Verification items for the finished model (mm, model axes). A direction names the side the tool comes from. Round coordinates to 2 decimals unless told otherwise and drop trailing zeros. Loops run counter-clockwise (first coordinate to the right, second up) from the corner with the lowest first, then second, coordinate; pieces in that order, holes last. Notation, with made-up numbers: (84.25, -18) - (120.25, -18) arc R22 cw to (120.25, 0) - close; hole circle Ø8 at (19.5, -17.75). An arc over 180 degrees is marked (long way). Use a Markdown table: item, result. Add a question column.
```python
from build123d import *

# Parameters (mm, degrees)
SKETCH1_W                                       = 55
SKETCH1_H                                       = 30
BOSS_EXTRUDE1_DEPTH                             = 3
SKETCH2_R                                       = 2.95
BOSS_EXTRUDE2_DEPTH                             = 4.9
SKETCH8_R                                       = 3.55
CUT_EXTRUDE2_DEPTH                              = 6
SKETCH10_W                                      = 3
SKETCH10_H                                      = 30
BOSS_EXTRUDE3_DEPTH                             = 6.5
BOSS_EXTRUDE3_DEPTH_BACK                        = 3
SKETCH11_W                                      = 3
SKETCH11_H                                      = 30
BOSS_EXTRUDE4_DEPTH                             = 6.5
BOSS_EXTRUDE4_DEPTH_BACK                        = 3
TAP_DRILL_FOR_M3X0_5_TAP1_AT_2_COUNT            = 2
TAP_DRILL_FOR_M3X0_5_TAP1_AT_2_PITCH            = 24
TAP_DRILL_FOR_M2_5X0_45_TAP2_D                  = 2.05
TAP_DRILL_FOR_M2_5X0_45_TAP2_DEPTH              = 6
TAP_DRILL_FOR_M2_5X0_45_TAP2_TIP                = 0.615882
SKETCH18_R                                      = 1.05
CUT_EXTRUDE4_DEPTH                              = 10
CIRPATTERN2_COUNT                               = 3
MIRROR3_COPY_1_SKETCH_R                         = 1.05
MIRROR3_COPY_1_DEPTH                            = 10
MIRROR3_COPY_2_SKETCH_R                         = 1.05
MIRROR3_COPY_2_DEPTH                            = 10
SKETCH21_W                                      = 55
SKETCH21_H                                      = 30
SKETCH21_R                                      = 4
CUT_EXTRUDE7_DEPTH                              = 0.5
SKETCH23_R                                      = 4
SKETCH23_R_2                                    = 3
CUT_EXTRUDE8_DEPTH                              = 0.1
CSK_FOR_M2_FLAT_HEAD_MACHINE_SCREW1_D           = 2.1
CSK_FOR_M2_FLAT_HEAD_MACHINE_SCREW1_DEPTH       = 9.5
CSK_FOR_M2_FLAT_HEAD_MACHINE_SCREW1_CSINK_D     = 3.5
CSK_FOR_M2_FLAT_HEAD_MACHINE_SCREW1_CSINK_ANGLE = 90
CSK_FOR_M2_FLAT_HEAD_MACHINE_SCREW1_TIP         = 0.630904
SKETCH25_W                                      = 55
SKETCH25_H                                      = 30
SKETCH25_R                                      = 3.55
SKETCH25_R_2                                    = 1.05
BOSS_EXTRUDE6_DEPTH                             = 0.5


with BuildPart() as part:
    # Sketch1 → Boss-Extrude1 (new body)
    with BuildSketch(Plane(origin=(0, 0, 0), x_dir=(1, 0, 0), z_dir=(0, 1, 0))):
        with Locations((27.5, 16)):
            Rectangle(SKETCH1_W, SKETCH1_H)
    extrude(amount=BOSS_EXTRUDE1_DEPTH)

    # Sketch2 → Boss-Extrude2 (add)
    with BuildSketch(Plane(origin=(0, 3, 0), x_dir=(1, 0, 0), z_dir=(0, 1, 0))):
        with Locations((27.5, 24.3)):
            Circle(SKETCH2_R)
    extrude(amount=BOSS_EXTRUDE2_DEPTH)

    # Sketch8 → Cut-Extrude2 (cut)
    with BuildSketch(Plane(origin=(0, 3, 0), x_dir=(1, 0, 0), z_dir=(0, 1, 0))):
        with Locations((43, 12.46784)):
            Circle(SKETCH8_R)
    cut_extrude2 = extrude(amount=-CUT_EXTRUDE2_DEPTH, mode=Mode.SUBTRACT)

    # Mirror1: Cut-Extrude2 across plane
    add(cut_extrude2.mirror(Plane(origin=(27.5, 0, 0), x_dir=(0, 0, 1), z_dir=(1, 0, 0))), mode=Mode.SUBTRACT)

    # Sketch10 → Boss-Extrude3 (add, two sides)
    with BuildSketch(Plane(origin=(0, 3, 0), x_dir=(1, 0, 0), z_dir=(0, 1, 0))) as boss_extrude3_sk:
        with Locations((56.5, 16)):
            Rectangle(SKETCH10_W, SKETCH10_H)
    extrude(amount=BOSS_EXTRUDE3_DEPTH)
    extrude(boss_extrude3_sk.sketch, amount=-BOSS_EXTRUDE3_DEPTH_BACK)

    # Sketch11 → Boss-Extrude4 (add, two sides)
    with BuildSketch(Plane(origin=(0, 3, 0), x_dir=(1, 0, 0), z_dir=(0, 1, 0))) as boss_extrude4_sk:
        with Locations((-1.5, 16)):
            Rectangle(SKETCH11_W, SKETCH11_H)
    extrude(amount=BOSS_EXTRUDE4_DEPTH)
    extrude(boss_extrude4_sk.sketch, amount=-BOSS_EXTRUDE4_DEPTH_BACK)

    # Sketch12 → Tap Drill for M3x0.5 Tap1 (revolve, cut)
    with BuildSketch(Plane(origin=(-3, 6.5, -28), x_dir=(0, 0, 1), z_dir=(0, 1, 0))):
        Polygon((0, 0), (0, 10.751076), (1.25, 10), (1.25, 0), align=None)
    tap_drill_for_m3x0_5_tap1 = revolve(axis=Axis((-9.35, 6.5, -28), (1, 0, 0)), mode=Mode.SUBTRACT)

    # Tap Drill for M3x0.5 Tap1 at 2: Tap Drill for M3x0.5 Tap1 ×2
    with Locations(*[(0, 0, i * TAP_DRILL_FOR_M3X0_5_TAP1_AT_2_PITCH) for i in range(1, TAP_DRILL_FOR_M3X0_5_TAP1_AT_2_COUNT)]):
        add(tap_drill_for_m3x0_5_tap1, mode=Mode.SUBTRACT)

    # Mirror2: Tap Drill for M3x0.5 Tap1 across plane
    add(tap_drill_for_m3x0_5_tap1.mirror(Plane(origin=(27.5, 0, 0), x_dir=(0, 0, 1), z_dir=(1, 0, 0))), mode=Mode.SUBTRACT)

    # Mirror2 copy 1 sketch → Mirror2 copy 1 (revolve, cut)
    with BuildSketch(Plane(origin=(58, 6.5, -4), x_dir=(0, 0, 1), z_dir=(0, 1, 0))):
        Polygon((0, 0), (0, -10.751076), (1.25, -10), (1.25, 0), align=None)
    revolve(axis=Axis((64.35, 6.5, -4), (1, 0, 0)), mode=Mode.SUBTRACT)

    # Tap Drill for M2.5x0.45 Tap2
    with Locations(Plane(origin=(0, 7.9, 0), x_dir=(1, 0, 0), z_dir=(0, 1, 0))):
        with Locations((27.5, 24.3)):
            Hole(TAP_DRILL_FOR_M2_5X0_45_TAP2_D / 2, depth=TAP_DRILL_FOR_M2_5X0_45_TAP2_DEPTH)
            with Locations((0, 0, -(TAP_DRILL_FOR_M2_5X0_45_TAP2_DEPTH + TAP_DRILL_FOR_M2_5X0_45_TAP2_TIP / 2))):  # 118° drill point
                Cone(0, TAP_DRILL_FOR_M2_5X0_45_TAP2_D / 2, TAP_DRILL_FOR_M2_5X0_45_TAP2_TIP, mode=Mode.SUBTRACT)

    # Sketch18 → Cut-Extrude4 (cut)
    with BuildSketch(Plane(origin=(0, 3, 0), x_dir=(1, 0, 0), z_dir=(0, 1, 0))):
        with Locations((12, 18.46784)):
            Circle(SKETCH18_R)
    cut_extrude4 = extrude(amount=-CUT_EXTRUDE4_DEPTH, mode=Mode.SUBTRACT)

    # CirPattern2: Cut-Extrude4 ×3 about axis
    cirpattern2_axis = Axis((12, 0, -12.46784), (0, 1, 0))
    for i in range(1, CIRPATTERN2_COUNT):
        add(cut_extrude4.rotate(cirpattern2_axis, i * 360 / CIRPATTERN2_COUNT), mode=Mode.SUBTRACT)

    # Mirror3: Cut-Extrude4 across plane
    add(cut_extrude4.mirror(Plane(origin=(27.5, 0, 0), x_dir=(0, 0, 1), z_dir=(1, 0, 0))), mode=Mode.SUBTRACT)

    # Mirror3 copy 1 sketch → Mirror3 copy 1 (cut)
    with BuildSketch(Plane(origin=(26.202533, 3, -8.309456), x_dir=(0.5, 0, -0.866025), z_dir=(0, 1, 0))):
        with Locations((12, -18.46784)):
            Circle(MIRROR3_COPY_1_SKETCH_R)
    extrude(amount=-MIRROR3_COPY_1_DEPTH, mode=Mode.SUBTRACT)

    # Mirror3 copy 2 sketch → Mirror3 copy 2 (cut)
    with BuildSketch(Plane(origin=(47.797467, 3, -29.094065), x_dir=(0.5, 0, 0.866025), z_dir=(0, 1, 0))):
        with Locations((12, -18.46784)):
            Circle(MIRROR3_COPY_2_SKETCH_R)
    extrude(amount=-MIRROR3_COPY_2_DEPTH, mode=Mode.SUBTRACT)

    # Sketch21 → Cut-Extrude7 (cut)
    with BuildSketch(Plane(origin=(0, 3, 0), x_dir=(1, 0, 0), z_dir=(0, 1, 0))):
        with Locations((27.5, 16)):
            Rectangle(SKETCH21_W, SKETCH21_H)
        with Locations((27.5, 24.3)):
            Circle(SKETCH21_R, mode=Mode.SUBTRACT)
    extrude(amount=-CUT_EXTRUDE7_DEPTH, mode=Mode.SUBTRACT)

    # Sketch23 → Cut-Extrude8 (cut)
    with BuildSketch(Plane(origin=(0, 3, 0), x_dir=(1, 0, 0), z_dir=(0, 1, 0))):
        with Locations((27.5, 24.3)):
            Circle(SKETCH23_R)
        with Locations((27.5, 24.3)):
            Circle(SKETCH23_R_2, mode=Mode.SUBTRACT)
    extrude(amount=-CUT_EXTRUDE8_DEPTH, mode=Mode.SUBTRACT)

    # CSK for M2 Flat Head Machine Screw1
    with Locations(Plane(origin=(43, 2.5, -18.46784), x_dir=(0, 0, 1), z_dir=(0, 1, 0))):
        with Locations((0, 0), (9, 5.196152), (9, -5.196152), (9, -25.803848), (0, -31), (9, -36.196152)):
            CounterSinkHole(CSK_FOR_M2_FLAT_HEAD_MACHINE_SCREW1_D / 2, CSK_FOR_M2_FLAT_HEAD_MACHINE_SCREW1_CSINK_D / 2, depth=CSK_FOR_M2_FLAT_HEAD_MACHINE_SCREW1_DEPTH, counter_sink_angle=CSK_FOR_M2_FLAT_HEAD_MACHINE_SCREW1_CSINK_ANGLE)
            with Locations((0, 0, -(CSK_FOR_M2_FLAT_HEAD_MACHINE_SCREW1_DEPTH + CSK_FOR_M2_FLAT_HEAD_MACHINE_SCREW1_TIP / 2))):  # 118° drill point
                Cone(0, CSK_FOR_M2_FLAT_HEAD_MACHINE_SCREW1_D / 2, CSK_FOR_M2_FLAT_HEAD_MACHINE_SCREW1_TIP, mode=Mode.SUBTRACT)

    # Sketch25 → Boss-Extrude6 (add)
    with BuildSketch(Plane(origin=(0, 0, 0), x_dir=(-1, 0, 0), z_dir=(0, -1, 0))):
        with Locations((-27.5, 16)):
            Rectangle(SKETCH25_W, SKETCH25_H)
        with Locations((-43, 12.46784)):
            Circle(SKETCH25_R, mode=Mode.SUBTRACT)
        with Locations((-48.196152, 9.46784)):
            Circle(SKETCH25_R_2, mode=Mode.SUBTRACT)
        with Locations((-43, 18.46784)):
            Circle(SKETCH25_R_2, mode=Mode.SUBTRACT)
        with Locations((-37.803848, 9.46784)):
            Circle(SKETCH25_R_2, mode=Mode.SUBTRACT)
        with Locations((-12, 12.46784)):
            Circle(SKETCH25_R, mode=Mode.SUBTRACT)
        with Locations((-17.196152, 9.46784)):
            Circle(SKETCH25_R_2, mode=Mode.SUBTRACT)
        with Locations((-12, 18.46784)):
            Circle(SKETCH25_R_2, mode=Mode.SUBTRACT)
        with Locations((-6.803848, 9.46784)):
            Circle(SKETCH25_R_2, mode=Mode.SUBTRACT)
    extrude(amount=BOSS_EXTRUDE6_DEPTH)


solid = part.part
```
Q1. Section check D-D on z = -4. Record the cut outline in (x, y).
Q2. Section check B-B on y = 6.5. Record the cut outline in (x, z) (3 decimals), plus the area to 3 significant figures.
Q3. Release check for a two-part mould opening along X. For faces 4 (the face through (55, 6, -16)), 5 (the face through (0, 6, -16)), 6 (the face through (-3, 5, -16)), 7 (the face through (56.521, 6.979, -26.845)) record: +X half, -X half, draft (parallel to the pull), parting line (faces both ways), or undercut.
Q4. Go/stop test with flat-tipped pins: pin 1 Ø4 at (x, z) = (29.5, -24.5) entering from +Y; pin 2 Ø6 at (x, y) = (39.5, 4.5) entering from +Z; pin 3 Ø1.8 at (x, z) = (27.5, -24.3) entering from +Y; pin 4 Ø8 at (x, z) = (43, -12.47) entering from +Y. Record where each tip stops, or that it passes through.
Q5. Section check C-C on x = 12. Record the cut outline in (y, z), plus the area to 3 significant figures.
Q6. Thickness scan on line 1 along Z through (x, y) = (12, 1.05); line 2 along X through (y, z) = (7.5, -11); line 3 along Y through (x, z) = (2.5, -24.5). Record the ranges inside material, lowest first.
Q7. Section check A-A on y = 3.75. Record the cut outline in (x, z) (3 decimals).
Q8. Set-up check for faces 1 (the face through (-1.521, 6.979, -26.845)), 2 (the face through (-2, 0, -16)), 3 (the face through (27, 7.9, -23)): record each of +Z, -Z, +X, -X, +Y, -Y from which the full face is reachable in a straight line by a thin tool's end or side.
Determined:
| question | item | result |
|---|---|---|
| 1 | outline | (-3, 0) - (0, 0) - (0, -0.5) - (55, -0.5) - (55, 0) - (58, 0) - (58, 5.25) - (55, 5.25) - (55, 2.5) - (0, 2.5) - (0, 5.25) - (-3, 5.25) - close; (-3, 7.75) - (0, 7.75) - (0, 9.5) - (-3, 9.5) - close; (55, 7.75) - (58, 7.75) - (58, 9.5) - (55, 9.5) - close |
| 2 | outline | (-3, -31) - (0, -31) - (0, -29.25) - (-3, -29.25) - close; (-3, -26.75) - (0, -26.75) - (0, -5.25) - (-3, -5.25) - close; (-3, -2.75) - (0, -2.75) - (0, -1) - (-3, -1) - close; circle Ø5.9 at (27.5, -24.3); (55, -31) - (58, -31) - (58, -29.25) - (55, -29.25) - close; (55, -26.75) - (58, -26.75) - (58, -5.25) - (55, -5.25) - close; (55, -2.75) - (58, -2.75) - (58, -1) - (55, -1) - close; hole circle Ø2.05 at (27.5, -24.3) |
| 2 | area | 174 mm² |
| 3 | face 4 | undercut |
| 3 | face 5 | undercut |
| 3 | face 6 | -X half |
| 3 | face 7 | draft |
| 4 | pin 1 | stops at y = 7.9 |
| 4 | pin 2 | stops at z = -1 |
| 4 | pin 3 | stops at y = 1.82 |
| 4 | pin 4 | stops at y = 2.5 |
| 5 | outline | (-0.5, -31) - (2.5, -31) - (2.5, -20.22) - (1.8, -19.52) - (-0.5, -19.52) - close; (-0.5, -17.42) - (1.8, -17.42) - (2.5, -16.72) - (2.5, -16.02) - (-0.5, -16.02) - close; (-0.5, -8.92) - (2.5, -8.92) - (2.5, -1) - (-0.5, -1) - close |
| 5 | area | 61.9 mm² |
| 6 | line 1 | z = -31 to -19.52, -17.42 to -16.02, -8.92 to -1 |
| 6 | line 2 | x = -3 to 0, 55 to 58 |
| 6 | line 3 | y = -0.5 to 2.5 |
| 7 | outline | (-3, -31) - (0, -31) - (0, -1) - (-3, -1) - close; circle Ø5.9 at (27.5, -24.3); (55, -31) - (58, -31) - (58, -1) - (55, -1) - close; hole circle Ø2.05 at (27.5, -24.3) |
| 8 | face 1 | -X |
| 8 | face 2 | +Z, -Z, -X, -Y |
| 8 | face 3 | +Z, -Z, +Y |
